```python
from build123d import *

# Parameters (mm, degrees)
BOSS_EXTRUDE1_START = -10
SKETCH1_R           = 3
SKETCH1_R_2         = 2
BOSS_EXTRUDE1_DEPTH = 5


with BuildPart() as part:
    # Sketch1 → Boss-Extrude1 (new body)
    with BuildSketch(Plane.XY.offset(BOSS_EXTRUDE1_START)):
        with BuildLine():
            Line((-125.350212025, 161.26892377), (-79.387545438, 161.26892377))
            ThreePointArc((-79.387545438, 161.26892377), (-74.748731312, 158.134775723), (-75.92540928, 152.661485175))
            Line((-75.92540928, 152.661485175), (-97.52188811, 131.934881446))
            ThreePointArc((-97.52188811, 131.934881446), (-102.368878731, 129.98529548), (-107.215869353, 131.934881446))
            Line((-107.215869353, 131.934881446), (-128.812348183, 152.661485175))
            ThreePointArc((-128.812348183, 152.661485175), (-129.98902615, 158.134775723), (-125.350212025, 161.26892377))
        make_face()
        with Locations((-102.368878731, 136.98529548)):
            Circle(SKETCH1_R, mode=Mode.SUBTRACT)
        with Locations((-79.387545438, 156.26892377)):
            Circle(SKETCH1_R_2, mode=Mode.SUBTRACT)
        with Locations((-125.350212025, 156.26892377)):
            Circle(SKETCH1_R_2, mode=Mode.SUBTRACT)
    extrude(amount=-BOSS_EXTRUDE1_DEPTH)


solid = part.part
```
Work out the finished part from the listing and answer in its coordinate system (mm). Coordinates: 2 decimals unless noted, no trailing zeros. Write each loop counter-clockwise with the first axis right and the second up, starting at its lowest first coordinate (ties: lowest second). Pieces come first, ordered by that corner, then holes. Notation, with made-up numbers: (-19, 37) - (4, 37) arc R15 cw to (4, 59) - close; hole circle Ø2 at (5, -36.5). An arc over 180 degrees is marked (long way). Answer as a JSON object with one key per item and string values.
Q1. Consider L1, parallel to X at y = 156.5, z = -12.35; L2, parallel to X at y = 158, z = -11.7; L3, parallel to X at y = 136, z = -11. Determine where each line is inside the solid, lowest interval first. Write a range as from..to.
Results list:
{"L1": "x = -130.34..-127.34, -123.36..-81.37, -77.4..-74.39", "L2": "x = -130.04..-126.35, -124.35..-80.39, -78.39..-74.7", "L3": "x = -111.45..-105.2, -99.54..-93.29"}
Q2. Given pin 1 Ø2.5 at (x, y) = (-125.35, 156.27) entering from -Z; pin 2 Ø3 at (y, z) = (146, -13.5) entering from +X, each flat-ended and moving along its own axis, determine where each tip first touches the part or whether it passes through.
Results list:
{"pin 1": "passes through", "pin 2": "stops at x = -81.3"}
Q3. Find section D-D (y = 136). Write down the section's boundary in (x, z), plus the area to 3 significant figures.
Results list:
{"outline": "(-111.45, -15) - (-105.2, -15) - (-105.2, -10) - (-111.45, -10) - close; (-99.54, -15) - (-93.29, -15) - (-93.29, -10) - (-99.54, -10) - close", "area": "62.5 mm^2"}
Q4. Find section B-B (x = -100.5). Write down the section's boundary in (y, z), plus the area to 3 significant figures.
Results list:
{"outline": "(130.24, -15) - (134.64, -15) - (134.64, -10) - (130.24, -10) - close; (139.33, -15) - (161.27, -15) - (161.27, -10) - (139.33, -10) - close", "area": "132 mm^2"}
Q5. Find section A-A (y = 155). Write down the section's boundary in (x, z), plus the area to 3 significant figures.
Results list:
{"outline": "(-130.19, -15) - (-126.9, -15) - (-126.9, -10) - (-130.19, -10) - close; (-123.8, -15) - (-80.93, -15) - (-80.93, -10) - (-123.8, -10) - close; (-77.84, -15) - (-74.55, -15) - (-74.55, -10) - (-77.84, -10) - close", "area": "247 mm^2"}
Q6. Find section C-C (z = -11.75). Write down the section's boundary in (x, y).
Results list:
{"outline": "(-128.81, 152.66) - (-107.22, 131.93) arc R7 ccw to (-97.52, 131.93) - (-75.93, 152.66) arc R5 ccw to (-79.39, 161.27) - (-125.35, 161.27) arc R5 ccw to start; hole circle Ø4 at (-125.35, 156.27); hole circle Ø6 at (-102.37, 136.99); hole circle Ø4 at (-79.39, 156.27)"}
Q7. For a pull along Y with two mould halves and no side action, classify faces 1 (the cylindrical face through (-104.58, 139.01, -12.46)), 2 (the cylindrical face through (-130.02, 158.06, -12.46)), 3 (the flat face through (-102, 149, -10)) as pulls with the +Y half, pulls with the -Y half, needs draft (parallel to the pull), parting line crosses it, or undercut.
Results list:
{"face 1": "undercut", "face 2": "parting line crosses it", "face 3": "needs draft"}
